Verification items for this drawing (mm, ordinates from the low corner). Round coordinates to 2 decimals unless told otherwise and drop trailing zeros. Write each loop counter-clockwise with the first axis right and the second up, starting at its lowest first coordinate (ties: lowest second). Pieces come first, ordered by that corner, then holes.
Item 1: Scan lines: probe 1 along Z at (x, y) = (30.43, 1.2) (3 decimals); probe 2 along Z at (x, y) = (26, 0.6). Record each from-to range of solid material in increasing order.
Item 2: Cross-section at B-B (y = 1.1). Enter the section's corners in (x, z) (3 decimals), then the cut area to 3 significant figures.
Item 3: Cross-section at A-A (x = 30.43). Enter the section's corners in (y, z) (3 decimals).
Item 4: Cross-section at C-C (z = 37). Enter the section's corners in (x, y).
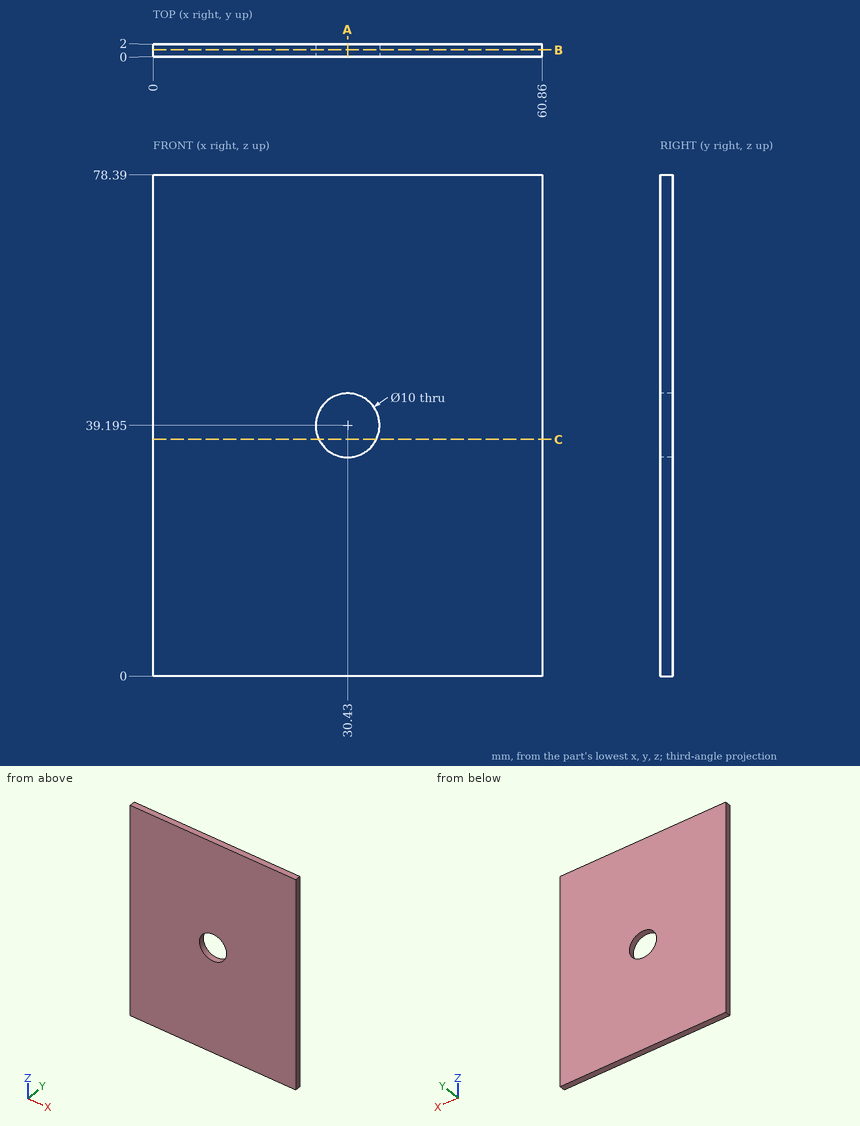
Resolved:
1. probe 1: z = 0 to 34.195, 44.195 to 78.39
1. probe 2: z = 0 to 36.88, 41.51 to 78.39
2. outline: (0, 0) - (60.86, 0) - (60.86, 78.39) - (0, 78.39) - close; hole circle Ø10 at (30.43, 39.195)
2. area: 4,690 mm2
3. outline: (0, 0) - (2, 0) - (2, 34.195) - (0, 34.195) - close; (0, 44.195) - (2, 44.195) - (2, 78.39) - (0, 78.39) - close
4. outline: (0, 0) - (25.94, 0) - (25.94, 2) - (0, 2) - close; (34.92, 0) - (60.86, 0) - (60.86, 2) - (34.92, 2) - close
